Check sheet for the drawn part. Datum: minimum x, y, z corner. Units: mm. Round coordinates to 2 decimals unless told otherwise and drop trailing zeros. Order: outer loops, then holes, each group sorted by start corner. A loop starts at its lowest first (then second) coordinate and runs counter-clockwise, first axis right, second up.
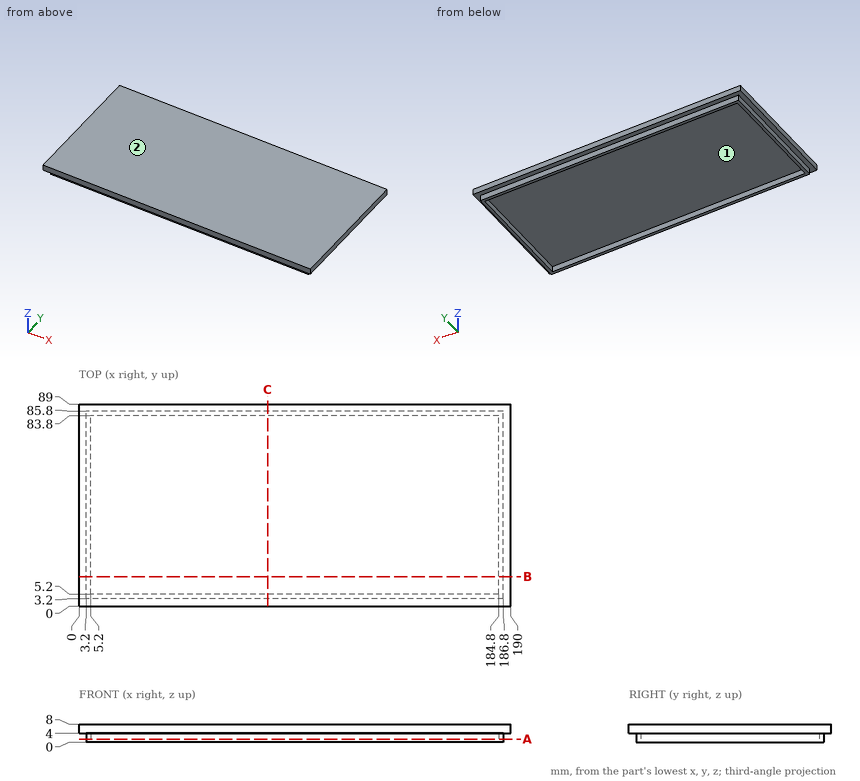
1) Draft check along Y on the marked faces 1 and 2. Enter one of: pulls with the +Y half, pulls with the -Y half, needs draft (parallel to the pull), parting line crosses it, or undercut.
2) Sectioned sample at B-B on y = 13. Record the cut outline in (x, z), and give its area (3 significant figures).
3) Sectioned sample at C-C on x = 83. Record the cut outline in (y, z).
4) Scan lines: line 1 (X direction, y = 64.5, z = 2.25); line 2 (Y direction, x = 174, z = 3); line 3 (Z direction, x = 31, y = 58.5). Record each from-to range of solid material in increasing order.
5) Sectioned sample at A-A on z = 1.5. Record the cut outline in (x, y).
6) Gauge pin test, flat ends, axial feed: pin 1 (3 mm diameter, centred on y = 32, z = 1.5, fed in from -X); pin 2 (3 mm diameter, centred on x = 92.5, z = 2, fed in from -Y); pin 3 (1.2 mm diameter, centred on x = 82.5, z = 2.5, fed in from +Y). Record the tip position at first contact, or that the pin passes through.
Values found:
1. face 1: undercut
1. face 2: needs draft
2. outline: (0, 4) - (3.2, 4) - (3.2, 0) - (5.2, 0) - (5.2, 4) - (184.8, 4) - (184.8, 0) - (186.8, 0) - (186.8, 4) - (190, 4) - (190, 8) - (0, 8) - close
2. area: 776 mm2
3. outline: (0, 4) - (3.2, 4) - (3.2, 0) - (5.2, 0) - (5.2, 4) - (83.8, 4) - (83.8, 0) - (85.8, 0) - (85.8, 4) - (89, 4) - (89, 8) - (0, 8) - close
4. line 1: x = 3.2 to 5.2, 184.8 to 186.8
4. line 2: y = 3.2 to 5.2, 83.8 to 85.8
4. line 3: z = 4 to 8
5. outline: (3.2, 3.2) - (186.8, 3.2) - (186.8, 85.8) - (3.2, 85.8) - close; hole (5.2, 5.2) - (184.8, 5.2) - (184.8, 83.8) - (5.2, 83.8) - close
6. pin 1: stops at x = 3.2
6. pin 2: stops at y = 3.2
6. pin 3: stops at y = 85.8
